Build history of the part. All positions in model axes, mm. Face numbers are marked on the shaded views. A direction names the side the tool comes from. Give positions to 0.01 mm unless a question says otherwise; leave off trailing zeros. Order: outer loops, then holes, each group sorted by start corner. A loop starts at its lowest first (then second) coordinate and runs counter-clockwise, first axis right, second up. Notation, with made-up numbers: (-28.5, 83) - (26.5, 83) arc R32 ccw to (26.5, 115) - close; hole circle Ø11 at (69, 66). An arc over 180 degrees is marked (long way). Answer in a Markdown table with one row per item.
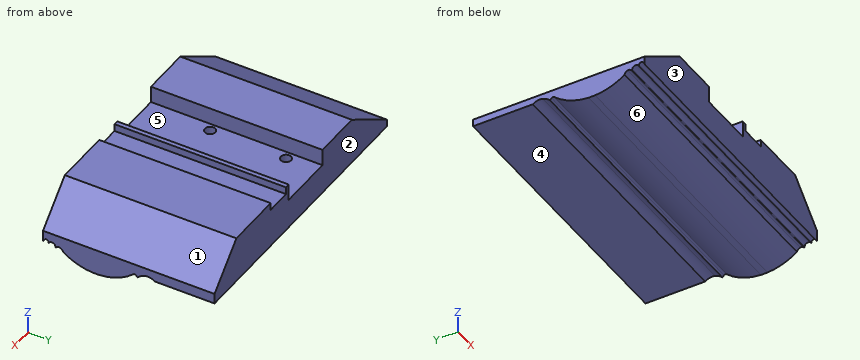
```python
from build123d import *

# Parameters (mm, degrees)
F1_DEPTH      = 68.072
F1_DEPTH_BACK = 68.072
F2_R          = 4.1275
F3_DEPTH      = 13.97
F5_DEPTH      = 228.6
F6_DEPTH      = 228.6


# Not quite as in the source:
# - a feature names something its author has since deleted; it is built from what else it names


with BuildPart() as f1:
    # F0 (on Front) → F1 (new body, two sides)
    with BuildSketch(Plane.XZ) as f1_sk:
        Polygon((-114.3, 0), (0, 0), (114.3, 0), (114.3, 20.32), (85.358465722, 48.9655555556), (39.892465722, 48.9655555556), (39.892465722, 43.1235555556), (19.572465722, 43.1235555556), (19.572465722, 48.9655555556), (15.940265722, 48.9655555556), (15.940265722, 35.7575555556), (-28.763734278, 35.7575555556), (-28.763734278, 48.9655555556), (-67.625734278, 48.9655555556), (-114.3, 17.78), align=None)
    extrude(amount=F1_DEPTH)
    extrude(f1_sk.sketch, amount=-F1_DEPTH_BACK)

    # F2 (on face) → F3 (cut)
    with BuildSketch(Plane.XY.offset(35.7575555556)):
        with Locations((-22.413734278, 42.926)):
            Circle(F2_R)
        with Locations((9.590265722, 42.926)):
            Circle(F2_R)
        with Locations((9.590265722, -17.272)):
            Circle(F2_R)
        with Locations((-22.413734278, -17.272)):
            Circle(F2_R)
    extrude(amount=-F3_DEPTH, mode=Mode.SUBTRACT)

    # F4 (on face) → F5 (cut)
    with BuildSketch(Plane.YZ.offset(114.3)):
        with BuildLine():
            ThreePointArc((-28.7846772927, 0), (-41.092836195, 2.5095205348), (-52.197, 8.382))
            ThreePointArc((-52.197, 8.382), (-53.0628215245, 10.1004124317), (-54.6900965273, 11.1273322254))
            ThreePointArc((-54.6900965273, 11.1273322254), (-55.6077664174, 11.233907182), (-56.5009973943, 10.9980795532))
            ThreePointArc((-56.5009973943, 10.9980795532), (-57.2399299218, 10.5397598563), (-57.8612, 9.9314))
            ThreePointArc((-57.8612, 9.9314), (-58.0475109479, 9.8713617946), (-58.1624396145, 10.0298160687))
            Line((-58.1624396145, 10.0298160687), (-58.2733862102, 10.82482934))
            ThreePointArc((-58.2733862102, 10.82482934), (-60.2066850368, 13.0247678359), (-62.9914626479, 12.1179120615))
            Line((-62.9914626479, 12.1179120615), (-63.4766221046, 11.5155344829))
            Line((-63.4766221046, 11.5155344829), (-63.6741071939, 12.5305661932))
            ThreePointArc((-63.6741071939, 12.5305661932), (-65.141327886, 13.96093331), (-66.995896399, 13.0895767361))
            Line((-66.995896399, 13.0895767361), (-68.072, 11.2702753395))
            Line((-68.072, 11.2702753395), (-68.072, 0))
            Line((-68.072, 0), (-28.7846772927, 0))
        make_face()
    extrude(amount=-F5_DEPTH, mode=Mode.SUBTRACT)

    # F4 (on face) → F6 (cut)
    with BuildSketch(Plane.YZ.offset(114.3)):
        with BuildLine():
            ThreePointArc((3.5306, 11.43), (-9.0647706891, 3.3847479258), (-23.622, 0))
            Line((-23.622, 0), (68.072, 0))
            Line((68.072, 0), (68.072, 12.065))
            Line((68.072, 12.065), (20.6756, 12.065))
            ThreePointArc((20.6756, 12.065), (16.8687140076, 13.8395100393), (12.6746, 13.6144))
            ThreePointArc((12.6746, 13.6144), (9.5960531105, 12.2103950232), (6.985, 10.0584))
            Line((6.985, 10.0584), (5.6642, 11.43))
            ThreePointArc((5.6642, 11.43), (4.5974, 11.8463817681), (3.5306, 11.43))
        make_face()
    extrude(amount=-F6_DEPTH, mode=Mode.SUBTRACT)


solid = f1.part
```
1. Cut at D-D on y = -50. Write the cut outline in (x, z), and give its area (3 significant figures).
Check result:
| item | result |
|---|---|
| outline | (-114.3, 6.88) - (114.3, 6.88) - (114.3, 20.32) - (85.36, 48.97) - (39.89, 48.97) - (39.89, 43.12) - (19.57, 43.12) - (19.57, 48.97) - (15.94, 48.97) - (15.94, 35.76) - (-28.76, 35.76) - (-28.76, 48.97) - (-67.63, 48.97) - (-114.3, 17.78) - close |
| area | 7,770 mm² |
2. Cut at A-A on x = 65.5. Write the cut outline in (y, z) (3 decimals), and give its area (3 significant figures).
Check result:
| item | result |
|---|---|
| outline | (-68.072, 11.27) - (-66.996, 13.09) arc R1.799 cw to (-63.674, 12.531) - (-63.477, 11.516) - (-62.991, 12.118) arc R2.663 cw to (-58.273, 10.825) - (-58.162, 10.03) arc R0.167 ccw to (-57.861, 9.931) arc R3.965 cw to (-56.501, 10.998) arc R2.486 cw to (-54.69, 11.127) arc R3.6 cw to (-52.197, 8.382) arc R44.174 ccw to (-28.785, 0) - (-23.622, 0) arc R44.174 ccw to (3.531, 11.43) arc R1.575 cw to (5.664, 11.43) - (6.985, 10.058) arc R12.979 cw to (12.675, 13.614) arc R8.661 cw to (20.676, 12.065) - (68.072, 12.065) - (68.072, 48.966) - (-68.072, 48.966) - close |
| area | 5,510 mm² |
3. Cut at C-C on y = 30.5. Write the cut outline in (x, z) (3 decimals), and give its area (3 significant figures).
Check result:
| item | result |
|---|---|
| outline | (-114.3, 12.065) - (114.3, 12.065) - (114.3, 20.32) - (85.358, 48.966) - (39.892, 48.966) - (39.892, 43.124) - (19.572, 43.124) - (19.572, 48.966) - (15.94, 48.966) - (15.94, 35.758) - (-28.764, 35.758) - (-28.764, 48.966) - (-67.626, 48.966) - (-114.3, 17.78) - close |
| area | 6,580 mm² |
4. Two-plate mould, pull along Y, no slides. Class the marked faces 1, 2 and 3: +Y half, -Y half, draft (parallel to the pull), parting line (faces both ways), or undercut.
Check result:
| item | result |
|---|---|
| face 1 | draft |
| face 2 | +Y half |
| face 3 | -Y half |
5. Which spindle directions (+Z, -Z, +X, -X, +Y, -Y) get a long thin tool onto all of the face, cutting with end or side? Do the marked faces 4, 5 and 6. Say none if no direction does.
Check result:
| item | result |
|---|---|
| face 4 | -Z, +X, -X, +Y |
| face 5 | +Z, +Y, -Y |
| face 6 | -Z, +X, -X, -Y |
6. Drop flat-ended pins along their axis: P1, Ø6.5, axis at x = 8, y = 42.5, coming from the +Z side; P2, Ø4, axis at x = -22.5, y = 43, coming from the +Z side; P3, Ø5, axis at y = -18.5, z = 39, coming from the -X side. Give the stop position or say it passes through.
Check result:
| item | result |
|---|---|
| P1 | stops at z = 35.76 |
| P2 | stops at z = 21.79 |
| P3 | stops at x = -86.28 |
7. Probe line 1 (X direction, y = -23, z = 46); line 2 (X direction, y = -52, z = 45.5); line 3 (Z direction, x = -53.5, y = 5). List the from-to ranges inside material, lowest first.
Check result:
| item | result |
|---|---|
| line 1 | x = -72.06 to -28.76, 15.94 to 19.57, 39.89 to 88.35 |
| line 2 | x = -72.81 to -28.76, 15.94 to 19.57, 39.89 to 88.86 |
| line 3 | z = 11.79 to 48.97 |
8. Cut at B-B on z = 45.5. Write the cut outline in (x, y).
Check result:
| item | result |
|---|---|
| outline | (-72.81, -68.07) - (-28.76, -68.07) - (-28.76, 68.07) - (-72.81, 68.07) - close; (15.94, -68.07) - (19.57, -68.07) - (19.57, 68.07) - (15.94, 68.07) - close; (39.89, -68.07) - (88.86, -68.07) - (88.86, 68.07) - (39.89, 68.07) - close |
